Could you check a few things on this model? Use its own coordinates, in mm. Face numbers are marked on the shaded views. A direction names the side the tool comes from. Give positions to 0.01 mm unless a question says otherwise; leave off trailing zeros. Answer as CSV lines item,"result". Start each with the question number.
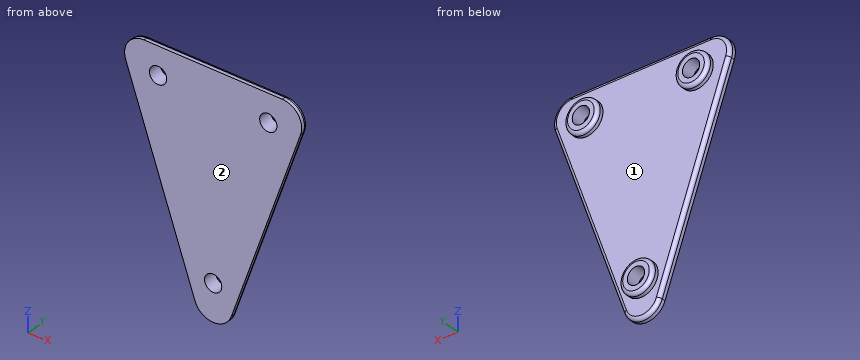
from build123d import *

# Parameters (mm, degrees)
BOSS_EXTRUDE1_DEPTH     = 1
BOSS_EXTRUDE3_START     = 1
SKETCH2_R               = 2.425
BOSS_EXTRUDE3_DEPTH     = 1
SKETCH3_R               = 1.25
CUT_EXTRUDE2_DEPTH      = 3
CUT_EXTRUDE2_DEPTH_BACK = 1
FILLET2_R               = 2.8
FILLET3_R               = 0.5


with BuildPart() as part:
    # Sketch1 → Boss-Extrude1 (new body)
    with BuildSketch(Plane(origin=(0, 0, 0), x_dir=(1, 0, 0), z_dir=(0, 1, 0))):
        Polygon((14, 0), (-14, 0), (0, 40), align=None)
    extrude(amount=BOSS_EXTRUDE1_DEPTH)

    # Sketch2 → Boss-Extrude3 (add)
    with BuildSketch(Plane(origin=(0, 0, 0), x_dir=(1, 0, 0), z_dir=(0, 1, 0)).offset(BOSS_EXTRUDE3_START)):
        with Locations((-8, 4)):
            Circle(SKETCH2_R)
        with Locations((0, 29)):
            Circle(SKETCH2_R)
        with Locations((8, 4)):
            Circle(SKETCH2_R)
    extrude(amount=BOSS_EXTRUDE3_DEPTH)

    # Sketch3 → Cut-Extrude2 (cut, two sides)
    with BuildSketch(Plane(origin=(0, 0, 0), x_dir=(1, 0, 0), z_dir=(0, 1, 0))) as cut_extrude2_sk:
        with Locations((0, 29)):
            Circle(SKETCH3_R)
        with Locations((-8, 4)):
            Circle(SKETCH3_R)
        with Locations((8, 4)):
            Circle(SKETCH3_R)
    extrude(amount=CUT_EXTRUDE2_DEPTH, mode=Mode.SUBTRACT)
    extrude(cut_extrude2_sk.sketch, amount=-CUT_EXTRUDE2_DEPTH_BACK, mode=Mode.SUBTRACT)

    # Fillet2
    fillet2_edges = [part.edges().sort_by_distance(p)[0] for p in [
        (0, 0.5, -40),
        (14, 0.5, 0),
        (-14, 0.5, 0),
    ]]
    fillet(fillet2_edges, radius=FILLET2_R)

    # Fillet3
    fillet3_edges = [part.edges().sort_by_distance(p)[0] for p in [
        (-10.425, 2, -4),
        (-2.425, 2, -29),
        (5.575, 2, -4),
        (-7.669529991, 1, -18.087057169),
        (7.669529991, 1, -18.087057169),
        (0, 1, 0),
        (-12.337084869, 1, -1.179806698),
        (12.337084869, 1, -1.179806698),
        (0, 1, -34.32415196),
    ]]
    fillet(fillet3_edges, radius=FILLET3_R)


solid = part.part
1. Please list where these lines run through material, in increasing order: line 1 (X direction, y = 1.1, z = -4) (3 decimals); line 2 (Z direction, x = 0, y = 1.15) (3 decimals); line 3 (Z direction, x = 8, y = 1.55).
2. Will this pin go through, and if not, where does the flat tip stop? P1, Ø5, axis at x = 0.5, z = -20.5, coming from the +Y side.
3. On a 3-axis mill with a long thin cutter (end or side, diameter ignored), from which of +Z, -Z, +X, -X, +Y, -Y can I reach the whole of each face in a straight line? I mean the marked faces 1 and 2. Say none if no direction works.
Solutions:
1,line 1,"-10.425 to -9.25, -6.75 to -5.575, 5.575 to 6.75, 9.25 to 10.425"
1,line 2,"-31.425 to -30.25, -27.75 to -26.575"
1,line 3,"-6.42 to -5.25, -2.75 to -1.58"
2,P1,"y = 1"
3,face 1,"+Y"
3,face 2,"+Z, -Z, +X, -X, -Y"
